from build123d import *

# Parameters (mm, degrees)
EXTRUDE_THIN1_DEPTH = 252.9
SKETCH2_W           = 19.05
SKETCH2_H           = 25.4
CUT_EXTRUDE1_DEPTH  = 3.175


with BuildPart() as part:
    # Sketch1 → Extrude-Thin1 (new body)
    with BuildSketch(Plane(origin=(0, 0, 0), x_dir=(1, 0, 0), z_dir=(0, 1, 0))):
        Polygon((0, 25.4), (0, 0), (25.4, 0), (25.4, 25.4), (22.225, 25.4), (22.225, 3.175), (3.175, 3.175), (3.175, 25.4), align=None)
    extrude(amount=EXTRUDE_THIN1_DEPTH)

    # Sketch2 → Cut-Extrude1 (cut)
    with BuildSketch(Plane(origin=(0, 0, -3.175), x_dir=(-1, 0, 0), z_dir=(0, 0, -1))):
        with Locations((-12.7, 12.7)):
            Rectangle(SKETCH2_W, SKETCH2_H)
        with Locations((-12.7, 240.2)):
            Rectangle(SKETCH2_W, SKETCH2_H)
    extrude(amount=-CUT_EXTRUDE1_DEPTH, mode=Mode.SUBTRACT)


solid = part.part
Design review of the part built by this model. Coordinates are the model's own, in mm. A direction names the side the tool comes from. Round coordinates to 2 decimals unless told otherwise and drop trailing zeros. Loops run counter-clockwise (first coordinate to the right, second up) from the corner with the lowest first, then second, coordinate; pieces in that order, holes last. Notation, with made-up numbers: M 86.25,79.5 L 132.25,79.5 A13 ccw 132.25,101.5 Z; hole C 30,-36.5 d10. An arc over 180 degrees is marked long. Answer as a JSON object with one key per item and string values.
Item 1: We need section A-A on z = -12.25. Give the boundary of the cut face in (x, y) (3 decimals).
Answer sheet:
{"outline": "M 0,0 L 3.175,0 L 3.175,252.9 L 0,252.9 Z; M 22.225,0 L 25.4,0 L 25.4,252.9 L 22.225,252.9 Z"}
Item 2: We need section C-C on x = 13.75. Give the boundary of the cut face in (y, z) (3 decimals).
Answer sheet:
{"outline": "M 25.4,-3.175 L 227.5,-3.175 L 227.5,0 L 25.4,0 Z"}
Item 3: We need section B-B on y = 130.5. Give the boundary of the cut face in (x, z) (3 decimals), and give its area (3 significant figures).
Answer sheet:
{"outline": "M 0,-25.4 L 3.175,-25.4 L 3.175,-3.175 L 22.225,-3.175 L 22.225,-25.4 L 25.4,-25.4 L 25.4,0 L 0,0 Z", "area": "222 mm^2"}
Item 4: Machinability: for faces 1 (the flat face through (13, 125, 0)), 2 (the flat face through (13, 125, -3.175)), which of the approach directions +Z, -Z, +X, -X, +Y, -Y give a long, thin tool a straight path to every point of the face, cutting with its end or side? Answer none if there is none.
Answer sheet:
{"face 1": "+Z, +X, -X, +Y, -Y", "face 2": "-Z, +Y, -Y"}
Item 5: Wall thickness on L1, parallel to X at y = 171, z = -9 (3 decimals); L2, parallel to Z at x = 14, y = 126 (3 decimals): over which ranges is each line inside the solid? List them lowest first. Write a range as from..to.
Answer sheet:
{"L1": "x = 0..3.175, 22.225..25.4", "L2": "z = -3.175..0"}
Item 6: Clearance check with flat-ended pins moving along their axes: P1, Ø1.6, axis at x = 16.5, z = -1, coming from the +Y side; P2, Ø1, axis at x = 5.5, y = 44, coming from the -Z side (3 decimals); P3, Ø2.5, axis at x = 13, z = -2, coming from the -Y side. State where each tip first meets the part, or that it passes through.
Answer sheet:
{"P1": "stops at y = 227.5", "P2": "stops at z = -3.175", "P3": "stops at y = 25.4"}
Item 7: The part is to be moulded in two halves that separate along X. For faces 3 (the flat face through (0, 125, -13)), 4 (the flat face through (3.175, 125, -13)), 5 (the flat face through (25.4, 125, -13)), say which applies: pulls with the +X half, pulls with the -X half, needs draft (parallel to the pull), parting line crosses it, or undercut.
Answer sheet:
{"face 3": "pulls with the -X half", "face 4": "undercut", "face 5": "pulls with the +X half"}
